```python
from build123d import *
from OCP.BRepFilletAPI import BRepFilletAPI_MakeFillet

# Parameters (mm, degrees)
SKETCH1_R           = 3.175
BOSS_EXTRUDE1_DEPTH = 6
BOSS_EXTRUDE2_START = -3.81
SKETCH1_3_W         = 38.1
SKETCH1_3_H         = 5.999999938
BOSS_EXTRUDE2_DEPTH = 24.13
SKETCH3_R           = 1.25
CUT_EXTRUDE1_DEPTH  = 44.944503594
FILLET1_R1          = 2.54
FILLET1_R2          = 5.08


with BuildPart() as part:
    # Sketch1 → Boss-Extrude1 (new body)
    with BuildSketch(Plane(origin=(3.81, 0, 0), x_dir=(0, 0, -1), z_dir=(1, 0, 0))):
        Polygon((-19.05, 0), (-19.05, -10.16), (0, -25.4), (19.05, -10.16), (19.05, 0), align=None)
        with Locations((0, -16.51)):
            Circle(SKETCH1_R, mode=Mode.SUBTRACT)
    boss_extrude1 = extrude(amount=BOSS_EXTRUDE1_DEPTH)

    # Sketch1<3> → Boss-Extrude2 (add)
    with BuildSketch(Plane(origin=(3.81, 0, 0), x_dir=(0, 0, -1), z_dir=(1, 0, 0)).offset(BOSS_EXTRUDE2_START)):
        with Locations((0, 2.999999969)):
            Rectangle(SKETCH1_3_W, SKETCH1_3_H)
    boss_extrude2 = extrude(amount=BOSS_EXTRUDE2_DEPTH)

    # Sketch3 → Cut-Extrude1 (cut, through all)
    with BuildSketch(Plane(origin=(0, 5.999999938, 0), x_dir=(1, 0, 0), z_dir=(0, 1, 0))):
        with Locations(Location((17.78, 12.7, 0), (0, 0, 270))):
            Circle(SKETCH3_R)
        with Locations(Location((17.78, -12.7, 0), (0, 0, 90))):
            Circle(SKETCH3_R)
    cut_extrude1 = extrude(amount=-CUT_EXTRUDE1_DEPTH, mode=Mode.SUBTRACT)

    # Mirror2: Boss-Extrude2, Cut-Extrude1 across plane
    add(boss_extrude2.mirror(Plane(origin=(0, 0, 0), x_dir=(0, 0, 1), z_dir=(1, 0, 0))))
    add(cut_extrude1.mirror(Plane(origin=(0, 0, 0), x_dir=(0, 0, 1), z_dir=(1, 0, 0))), mode=Mode.SUBTRACT)

    # Mirror3: Boss-Extrude1 across plane
    add(boss_extrude1.mirror(Plane(origin=(0, 0, 0), x_dir=(0, 0, 1), z_dir=(1, 0, 0))))

    # Fillet1: one fillet with a radius per group of edges: ONE call of the kernel's fillet builder (fillet() takes one radius for all edges)
    fillet1_edges_1 = [part.edges().sort_by_distance(p)[0] for p in [
        (6.81, -10.16, 19.05),
        (6.81, -10.16, -19.05),
        (9.81, 0, 0),
        (24.13, 2.999999969, 19.05),
        (24.13, 2.999999969, -19.05),
        (-24.13, 2.999999969, -19.05),
        (-24.13, 2.999999969, 19.05),
        (-6.81, -10.16, -19.05),
        (-6.81, -10.16, 19.05),
        (-3.81, 0, 0),
        (-9.81, 0, 0),
        (3.81, 0, 0),
    ]]
    fillet1_edges_2 = [part.edges().sort_by_distance(p)[0] for p in [
        (6.81, -25.4, 0),
        (-6.81, -25.4, 0),
    ]]
    fillet1 = BRepFilletAPI_MakeFillet(part.part.solid().wrapped)
    for e in fillet1_edges_1:
        fillet1.Add(FILLET1_R1, e.wrapped)
    for e in fillet1_edges_2:
        fillet1.Add(FILLET1_R2, e.wrapped)
    add(Compound.cast(fillet1.Shape()), mode=Mode.REPLACE)


solid = part.part
```
The model under review builds one solid part; all positions refer to its coordinate system, in mm. A direction names the side the tool comes from. Round coordinates to 2 decimals unless told otherwise and drop trailing zeros. Order: outer loops, then holes, each group sorted by start corner. A loop starts at its lowest first (then second) coordinate and runs counter-clockwise, first axis right, second up.
Item 1: Add section C-C, the plane x = -9. State the section outline as (y, z) points (3 decimals).
Working result:
outline: (-22.861, -3.173) - (-10.923, -18.097) arc R2.54 ccw to (-8.939, -19.05) - (6, -19.05) - (6, 19.05) - (-8.939, 19.05) arc R2.54 ccw to (-10.923, 18.097) - (-22.861, 3.173) arc R5.08 ccw to start; hole circle Ø6.35 at (-16.51, 0)
Item 2: Machinability: for faces 1 (the cylindrical face through (3.046, -0.724, 0.267)), 2 (the flat face through (9.81, -11, 0)), 3 (the flat face through (0, 2, -19.05)), which of the approach directions +Z, -Z, +X, -X, +Y, -Y give a long, thin tool a straight path to every point of the face, cutting with its end or side? Answer none if there is none.
Working result:
face 1: +Z, -Z, -Y
face 2: +Z, -Z, +X, -Y
face 3: -Z, +X, -X, +Y, -Y
Item 3: Add section D-D, the plane x = 17.78. State the section outline as (y, z) points, and give its area (3 significant figures).
Working result:
outline: (0, -19.05) - (6, -19.05) - (6, -13.95) - (0, -13.95) - close; (0, -11.45) - (6, -11.45) - (6, 11.45) - (0, 11.45) - close; (0, 13.95) - (6, 13.95) - (6, 19.05) - (0, 19.05) - close
area: 199 mm2
Item 4: For pin 1 (4 mm diameter, centred on x = 17.78, z = -12.7, fed in from -Y); pin 2 (3 mm diameter, centred on x = -1, z = -15, fed in from -Y); pin 3 (2 mm diameter, centred on x = -6, z = 5.5, fed in from -Y), all flat-tipped, find the tip position at first contact; note any pin that passes through.
Working result:
pin 1: stops at y = 0
pin 2: stops at y = -0.32
pin 3: stops at y = -21.8
Item 5: Add section A-A, the plane z = 12.7. State the section outline as (x, y) points.
Working result:
outline: (-24.13, 0) - (-19.03, 0) - (-19.03, 6) - (-24.13, 6) - close; (-16.53, 0) - (-12.35, 0) arc R2.54 cw to (-9.81, -2.54) - (-9.81, -15.24) - (-3.81, -15.24) - (-3.81, -2.54) arc R2.54 cw to (-1.27, 0) - (1.27, 0) arc R2.54 cw to (3.81, -2.54) - (3.81, -15.24) - (9.81, -15.24) - (9.81, -2.54) arc R2.54 cw to (12.35, 0) - (16.53, 0) - (16.53, 6) - (-16.53, 6) - close; (19.03, 0) - (24.13, 0) - (24.13, 6) - (19.03, 6) - close
Item 6: Draft analysis for pull direction Z (two halves, no side actions). For faces 4 (the cylindrical face through (-23.406, 3.042, -18.286)), 5 (the cylindrical face through (-6.77, -19.61, 0.69)), 6 (the flat face through (-18, 0, 0)), state which applies: released by +Z, released by -Z, zero draft, split by the parting line, or undercut.
Working result:
face 4: released by -Z
face 5: undercut
face 6: zero draft
Item 7: To check wall thickness, follow probe 1 along X at (y, z) = (3.7, -12.7); probe 2 along Z at (x, y) = (-17.78, 4); probe 3 along X at (y, z) = (-7.25, 16). State the ranges of each line that lie inside material, in increasing order.
Working result:
probe 1: x = -24.13 to -19.03, -16.53 to 16.53, 19.03 to 24.13
probe 2: z = -19.05 to -13.95, -11.45 to 11.45, 13.95 to 19.05
probe 3: x = -9.81 to -3.81, 3.81 to 9.81
Item 8: Add section B-B, the plane y = -3.25. State the section outline as (x, z) points, and give its area (3 significant figures).
Working result:
outline: (-9.81, -19.05) - (-3.81, -19.05) - (-3.81, 19.05) - (-9.81, 19.05) - close; (3.81, -19.05) - (9.81, -19.05) - (9.81, 19.05) - (3.81, 19.05) - close
area: 457 mm2
